The listing builds one solid part. Answer for the finished solid, in the listing's coordinates (mm). Face numbers are marked on the shaded views. A direction names the side the tool comes from. Coordinates: 2 decimals unless noted, no trailing zeros. Write each loop counter-clockwise with the first axis right and the second up, starting at its lowest first coordinate (ties: lowest second). Pieces come first, ordered by that corner, then holes. Notation, with made-up numbers: M 24,3 L 80,3 A23 ccw 80,21 Z; hole C 80.25,37.5 d3. An arc over 180 degrees is marked long. Answer as CSV lines item,"result".
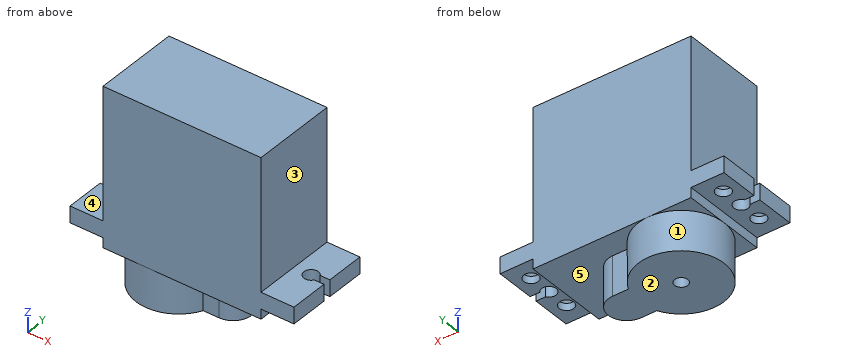
```python
from build123d import *

# Parameters (mm, degrees)
SKETCH_1_W          = 24
SKETCH_1_H          = 13
EXTRUDE_1_DEPTH     = 24
SKETCH_2_W          = 34
SKETCH_2_H          = 13
EXTRUDE_2_DEPTH     = 2.5
MM_13_D             = 2.2
MM_13_DEPTH         = 1.076990406
MM_13_TIP           = 0.923009594
CUT_EXTRUDE_1_DEPTH = 3.5
EXTRUDE_3_DEPTH     = 6
SKETCH_42_R         = 1
CUT_EXTRUDE_2_DEPTH = 4


with BuildPart() as part:
    # 草图1 → 凸台-拉伸1 (new body)
    with BuildSketch(Plane.XY):
        with Locations((12, 6.5)):
            Rectangle(SKETCH_1_W, SKETCH_1_H)
    extrude(amount=EXTRUDE_1_DEPTH)

    # 草图2 → 凸台-拉伸2 (add)
    with BuildSketch(Plane.XY.offset(1.5)):
        with Locations((12, 6.5)):
            Rectangle(SKETCH_2_W, SKETCH_2_H)
    extrude(amount=EXTRUDE_2_DEPTH)

    # 大小mm 暗销孔13
    with Locations(Plane(origin=(0, 0, 1.5), x_dir=(-1, 0, 0), z_dir=(0, 0, -1))):
        with Locations((2.6, 10), (2.6, 3), (-26.6, 10), (-26.6, 3)):
            Hole(MM_13_D / 2, depth=MM_13_DEPTH)
            with Locations((0, 0, -(MM_13_DEPTH + MM_13_TIP / 2))):  # 100° drill point
                Cone(0, MM_13_D / 2, MM_13_TIP, mode=Mode.SUBTRACT)

    # 草图6 → 切除-拉伸1 (cut)
    with BuildSketch(Plane.XY.offset(1.5)):
        with BuildLine():
            Line((-5, 7.074764733), (-3.537894185, 7.074764733))
            ThreePointArc((-3.537894185, 7.074764733), (-1.5, 6.5), (-3.537894185, 5.925235267))
            Line((-3.537894185, 5.925235267), (-5, 5.925235267))
            Line((-5, 5.925235267), (-5, 7.074764733))
        make_face()
        with BuildLine():
            Line((29, 5.925235267), (27.537894185, 5.925235267))
            ThreePointArc((27.537894185, 5.925235267), (25.5, 6.5), (27.537894185, 7.074764733))
            Line((27.537894185, 7.074764733), (29, 7.074764733))
            Line((29, 7.074764733), (29, 5.925235267))
        make_face()
    extrude(amount=CUT_EXTRUDE_1_DEPTH, mode=Mode.SUBTRACT)

    # 草图27 → 凸台-拉伸3 (add)
    with BuildSketch(Plane(origin=(0, 0, 0), x_dir=(-1, 0, 0), z_dir=(0, 0, -1))):
        with BuildLine():
            Line((-14.765807305, 3.7), (-12.36600375, 3.7))
            ThreePointArc((-12.36600375, 3.7), (0, 6.5), (-12.36600375, 9.3))
            Line((-12.36600375, 9.3), (-14.765807305, 9.3))
            ThreePointArc((-14.765807305, 9.3), (-17.565807305, 6.5), (-14.765807305, 3.7))
        make_face()
    extrude(amount=EXTRUDE_3_DEPTH)

    # 草图42 → 切除-拉伸2 (cut)
    with BuildSketch(Plane(origin=(0, 0, -6), x_dir=(-1, 0, 0), z_dir=(0, 0, -1))):
        with Locations((-6.5, 6.5)):
            Circle(SKETCH_42_R)
    extrude(amount=-CUT_EXTRUDE_2_DEPTH, mode=Mode.SUBTRACT)


solid = part.part
```
Q1. Find section A-A (z = 14.25). Give the vertices of the cut face in (x, y).
Output:
outline,"M 0,0 L 24,0 L 24,13 L 0,13 Z"
Q2. Find section B-B (y = 12.25). Give the vertices of the cut face in (x, z), and give its area (3 significant figures).
Output:
outline,"M -5,1.5 L 0,1.5 L 0,0 L 3.47,0 L 3.47,-6 L 9.53,-6 L 9.53,0 L 24,0 L 24,1.5 L 29,1.5 L 29,4 L 24,4 L 24,24 L 0,24 L 0,4 L -5,4 Z"
area,"637 mm2"
Q3. For the marked faces 1, 2, 3, 4 and 5, determine the directions among +Z, -Z, +X, -X, +Y, -Y from which every point of the face is accessible in a straight line to the end or side of a thin tool.
Output:
face 1,"-Z"
face 2,"-Z, +X, -X, +Y, -Y"
face 3,"+Z, +X, +Y, -Y"
face 4,"+Z, -X, +Y, -Y"
face 5,"-Z, +X"
Q4. Flat-ended cylindrical pins translate along their axes: pin 1 Ø1 at (y, z) = (7, 3) entering from -X; pin 2 Ø6.5 at (y, z) = (8, 18.5) entering from -X; pin 3 Ø1 at (x, y) = (17.5, 4) entering from -Z; pin 4 Ø2.5 at (x, y) = (-2.6, 10) entering from -Z. Find the tip coordinate at first contact, or state that the pin passes through.
Output:
pin 1,"x = -5"
pin 2,"x = 0"
pin 3,"z = 0"
pin 4,"z = 1.5"
Q5. Find section D-D (x = 21.5). Give the vertices of the cut face in (y, z), and give its area (3 significant figures).
Output:
outline,"M 0,0 L 13,0 L 13,24 L 0,24 Z"
area,"312 mm2"
Q6. Straight lines are drawn through the part: line 1 (X direction, y = 10, z = 2.2); line 2 (Y direction, x = 26.6, z = 2.4); line 3 (Y direction, x = 6.5, z = -2.9). For each, find the intervals that lie inside material, in ascending order.
Output:
line 1,"-5 to -3.7, -1.5 to 25.5, 27.7 to 29"
line 2,"0 to 1.9, 4.1 to 5.4, 7.6 to 8.9, 11.1 to 13"
line 3,"0 to 5.5, 7.5 to 13"
Q7. Find section C-C (x = 11.5). Give the vertices of the cut face in (y, z), and give its area (3 significant figures).
Output:
outline,"M 0,0 L 2.35,0 L 2.35,-6 L 10.65,-6 L 10.65,0 L 13,0 L 13,24 L 0,24 Z"
area,"362 mm2"
